Here's how the part is built. I have some questions about the finished solid (model axes, mm). A direction names the side the tool comes from. Give positions to 0.01 mm unless a question says otherwise; leave off trailing zeros. Loops run counter-clockwise (first coordinate to the right, second up) from the corner with the lowest first, then second, coordinate; pieces in that order, holes last. Notation, with made-up numbers: (79.5, 60.5) - (110.5, 60.5) arc R33 cw to (110.5, 95.5) - close; hole circle Ø7 at (27.5, 52). An arc over 180 degrees is marked (long way). Return JSON: item names as keys, results as strings. Group by question number.
(1) If we section it at A-A (y = -3): Please give me the cut outline in (x, z) (3 decimals).
(2) I need wall thicknesses on probe 1 along Y at (x, z) = (32, -15); probe 2 along X at (y, z) = (26, -7); probe 3 along X at (y, z) = (26.5, -7.9). Which ranges of each line are inside material? Lowest first, please. Write a range as [from, to].
(3) On a 3-axis mill with a long thin cutter (end or side, diameter ignored), from which of +Z, -Z, +X, -X, +Y, -Y can I reach the whole of each face in a straight line? I mean faces 5 (the flat face through (3, 11, 0)), 6 (the cylindrical face through (11.92, 25.93, -10.38)), 7 (the flat face through (23, 11, 5)), 8 (the flat face through (33.8, 25.9, -18.6)), 9 (the flat face through (22, 11, 14)). Say none if no direction works.
(4) If we section it at B-B (x = 33.5): Please give me the cut outline in (y, z), then the cut area to 3 significant figures.
(5) If we section it at C-C (y = 14.5): Please give me the cut outline in (x, z).
(6) For P1, Ø6.5, axis at x = 41, y = 6.5, coming from the -Z side; P2, Ø3, axis at x = 33, z = -7.9, coming from the -Y side; P3, Ø10.5, axis at x = 24.5, y = 9.5, coming from the -Z side, each with a flat end and sliding along its axis, tell me the tip position at first contact or that it passes through.
(7) If we mould it in two halves opening along X, with no side actions, what happens to faces 1 (the flat face through (0, 10, 1)), 2 (the flat face through (5.94, 10, 2)), 3 (the flat face through (42, 11, 0)), 4 (the flat face through (39.31, 10, 2))? For each: released by +X, released by -X, zero draft, split by the parting line, or undercut.
(8) If we section it at D-D (z = -23.5): Please give me the cut outline in (x, y), then the cut area to 3 significant figures.
```python
from build123d import *

# Parameters (mm, degrees)
SKETCH1_W           = 45.25
SKETCH1_H           = 21
BOSS_EXTRUDE1_DEPTH = 8
BOSS_EXTRUDE3_DEPTH = 10
BOSS_EXTRUDE4_DEPTH = 10
SKETCH5_W           = 45.25
SKETCH5_H           = 8
BOSS_EXTRUDE5_DEPTH = 10
SKETCH6_W           = 45.25
SKETCH6_H           = 8
BOSS_EXTRUDE6_DEPTH = 10
SKETCH7_W           = 33.369667902
SKETCH7_H           = 21
CUT_EXTRUDE1_DEPTH  = 5
SKETCH8_W           = 45.25
SKETCH8_H           = 41
BOSS_EXTRUDE7_DEPTH = 6
HOLE1_START         = -10
HOLE1_OUTLINE_R     = 2.5
HOLE1_DEPTH         = 41
HOLE2_START         = -10
HOLE2_OUTLINE_R     = 2.5
HOLE2_DEPTH         = 41


# Read off the part's stored shape, not the designer's step: Hole1, Hole2
with BuildPart() as part:
    # Sketch1 → Boss-Extrude1 (new body)
    with BuildSketch(Plane.XY):
        with Locations((22.625, 10.5)):
            Rectangle(SKETCH1_W, SKETCH1_H)
    extrude(amount=BOSS_EXTRUDE1_DEPTH)



with BuildPart() as body_2:
    # Sketch3 → Boss-Extrude3 (new body)
    with BuildSketch(Plane(origin=(0, 21, 0), x_dir=(1, 0, 0), z_dir=(0, 1, 0))):
        Polygon((45.25, 0), (0, 0), (0, 30.05), (22.625, 7.420166262), (45.25, 30.05), align=None)
    extrude(amount=BOSS_EXTRUDE3_DEPTH)


with BuildPart() as body_3:
    # Sketch4 → Boss-Extrude4 (new body)
    with BuildSketch(Plane.XZ):
        Polygon((0, 0), (45.25, 0), (45.25, -30.05), (22.625, -7.420166262), (0, -30.05), align=None)
    extrude(amount=BOSS_EXTRUDE4_DEPTH)


with BuildPart() as part_1:
    add(part.part)

    add(body_2.part)  # Boss-Extrude5 merges body 2
    # Sketch5 → Boss-Extrude5 (add)
    with BuildSketch(Plane(origin=(0, 21, 0), x_dir=(1, 0, 0), z_dir=(0, 1, 0))):
        with Locations((22.625, -4)):
            Rectangle(SKETCH5_W, SKETCH5_H)
    extrude(amount=BOSS_EXTRUDE5_DEPTH)


    add(body_3.part)  # Boss-Extrude6 merges body 3
    # Sketch6 → Boss-Extrude6 (add)
    with BuildSketch(Plane.XZ):
        with Locations((22.625, 4)):
            Rectangle(SKETCH6_W, SKETCH6_H)
    extrude(amount=BOSS_EXTRUDE6_DEPTH)

    # Sketch7 → Cut-Extrude1 (cut)
    with BuildSketch(Plane(origin=(0, 0, 0), x_dir=(-1, 0, 0), z_dir=(0, 0, -1))):
        with Locations((-22.625, 10.5)):
            Rectangle(SKETCH7_W, SKETCH7_H)
    extrude(amount=-CUT_EXTRUDE1_DEPTH, mode=Mode.SUBTRACT)

    # Sketch8 → Boss-Extrude7 (add)
    with BuildSketch(Plane.XY.offset(8)):
        with Locations((22.625, 10.5)):
            Rectangle(SKETCH8_W, SKETCH8_H)
    extrude(amount=BOSS_EXTRUDE7_DEPTH)

    # Hole1 outline → Hole1 (cut)
    with BuildSketch(Plane(origin=(0, 0, 0), x_dir=(1, 0, 0), z_dir=(0, 1, 0)).offset(HOLE1_START)):
        with Locations((33.003168971, 7.9)):
            Circle(HOLE1_OUTLINE_R)
    extrude(amount=HOLE1_DEPTH, mode=Mode.SUBTRACT)

    # Hole2 outline → Hole2 (cut)
    with BuildSketch(Plane(origin=(0, 0, 0), x_dir=(1, 0, 0), z_dir=(0, 1, 0)).offset(HOLE2_START)):
        with Locations((12.246831029, 7.9)):
            Circle(HOLE2_OUTLINE_R)
    extrude(amount=HOLE2_DEPTH, mode=Mode.SUBTRACT)


solid = part_1.part
```
Values:
{
 "1": {"outline": "(0, -30.05) - (22.625, -7.42) - (45.25, -30.05) - (45.25, 14) - (0, 14) - close; hole circle Ø5 at (12.247, -7.9); hole circle Ø5 at (33.003, -7.9)"},
 "2": {"probe 1": "[-10, 0], [21, 31]", "probe 2": "[0, 9.91], [14.58, 30.67], [35.34, 45.25]", "probe 3": "[0, 9.75], [14.75, 22.15], [23.1, 30.5], [35.5, 45.25]"},
 "3": {"face 5": "-Z, +X, -X", "face 6": "+Y, -Y", "face 7": "-Z", "face 8": "-Z, +Y, -Y", "face 9": "+Z, +X, -X, +Y, -Y"},
 "4": {"outline": "(-10, -18.3) - (0, -18.3) - (0, -10.35) - (-10, -10.35) - close; (-10, -5.45) - (0, -5.45) - (0, 5) - (21, 5) - (21, -5.45) - (31, -5.45) - (31, 14) - (-10, 14) - close; (21, -18.3) - (31, -18.3) - (31, -10.35) - (21, -10.35) - close", "area": "737 mm2"},
 "5": {"outline": "(0, 0) - (5.94, 0) - (5.94, 5) - (39.31, 5) - (39.31, 0) - (45.25, 0) - (45.25, 14) - (0, 14) - close"},
 "6": {"P1": "z = 0", "P2": "through", "P3": "z = 5"},
 "7": {"face 1": "released by -X", "face 2": "undercut", "face 3": "zero draft", "face 4": "undercut"},
 "8": {"outline": "(0, -10) - (6.55, -10) - (6.55, 0) - (0, 0) - close; (0, 21) - (6.55, 21) - (6.55, 31) - (0, 31) - close; (38.7, -10) - (45.25, -10) - (45.25, 0) - (38.7, 0) - close; (38.7, 21) - (45.25, 21) - (45.25, 31) - (38.7, 31) - close", "area": "262 mm2"}
}
